from build123d import *

# Parameters (mm, degrees)
SKETCH007_R                          = 3.25
EXTRUDE006_DEPTH                     = 10
SKETCH006_AS_DRAWN_R                 = 9
EXTRUDE005_DEPTH                     = 27
EXTRUDE005_ONTO_SKETCH006_ROLL_ANGLE = 90
SKETCH_R                             = 3.5
SKETCH_R_2                           = 1.75
EXTRUDE_DEPTH                        = 30
SKETCH001_AS_DRAWN_R                 = 12.5
EXTRUDE004_DEPTH                     = 50
EXTRUDE004_ONTO_SKETCH001_ROLL_ANGLE = 90
EXTRUDE002_DEPTH                     = 60
SKETCH003_AS_DRAWN_W                 = 50
SKETCH003_AS_DRAWN_H                 = 16
EXTRUDE003_DEPTH                     = 98
EXTRUDE003_ONTO_SKETCH003_ROLL_ANGLE = 90
CHAMFER_SIZE                         = 0.5


with BuildPart() as extrude006:
    # Sketch007 → Extrude006 (new body)
    with BuildSketch(Plane.XY):
        with Locations((-16, 45)):
            Circle(SKETCH007_R)
        with Locations((16, 45)):
            Circle(SKETCH007_R)
        with Locations((-16, 65)):
            Circle(SKETCH007_R)
        with Locations((16, 65)):
            Circle(SKETCH007_R)
    extrude(amount=EXTRUDE006_DEPTH)


with BuildPart() as extrude006_1:
    # Extrude006 placement: moved
    add(extrude006.part.moved(Location((0, 0, 7))))


with BuildPart() as extrude005:
    # Sketch006 as drawn → Extrude005 (new)
    with BuildSketch(Plane.XY):
        Circle(SKETCH006_AS_DRAWN_R)
    extrude(amount=-EXTRUDE005_DEPTH)


with BuildPart() as extrude005_1:
    # Extrude005 onto Sketch006 roll: moved
    add(extrude005.part.rotate(Axis((0, 0, 0), (1, 0, 0)), EXTRUDE005_ONTO_SKETCH006_ROLL_ANGLE))


with BuildPart() as extrude005_2:
    # Extrude005 onto Sketch006 placement: moved
    add(extrude005_1.part.moved(Location((0, 33, 0))))


with BuildPart() as extrude005_3:
    # Extrude005 placement: moved
    add(extrude005_2.part.moved(Location((0, -18, 0))))


with BuildPart() as sweep_body:
    # Sweep: sweep along a path in Sketch005
    with BuildLine(Plane.YZ) as sweep_path:
        Line((70, 40), (40, 40))
        Line((40, 40), (32.928932, 47.071068))
    # Sketch004 → Sweep (sweep)
    with BuildSketch(Plane.XZ.offset(-70)):
        Polygon((-12, 16), (12, 16), (14, 10), (21, 10), (21, 28), (-21, 28), (-21, 10), (-14, 10), align=None)
    sweep(path=sweep_path.line, transition=Transition.RIGHT)


with BuildPart() as extrude_body:
    # Sketch → Extrude (new body)
    with BuildSketch(Plane.XY):
        Circle(SKETCH_R)
        with Locations((-16, 45)):
            Circle(SKETCH_R_2)
        with Locations((-16, 65)):
            Circle(SKETCH_R_2)
        with Locations((16, 65)):
            Circle(SKETCH_R_2)
        with Locations((16, 45)):
            Circle(SKETCH_R_2)
        with BuildLine():
            ThreePointArc((-12.020815, -9.192388), (-12.020815, -12.020815), (-9.192388, -12.020815))
            Line((-9.192388, -12.020815), (-4.242641, -7.071068))
            ThreePointArc((-4.242641, -7.071068), (-4.242641, -4.242641), (-7.071068, -4.242641))
            Line((-12.020815, -9.192388), (-7.071068, -4.242641))
        make_face()
        with BuildLine():
            ThreePointArc((7.071068, -4.242641), (4.242641, -4.242641), (4.242641, -7.071068))
            Line((4.242641, -7.071068), (9.192388, -12.020815))
            ThreePointArc((9.192388, -12.020815), (12.020815, -12.020815), (12.020815, -9.192388))
            Line((7.071068, -4.242641), (12.020815, -9.192388))
        make_face()
        with BuildLine():
            ThreePointArc((4.242641, 7.071068), (4.242641, 4.242641), (7.071068, 4.242641))
            Line((7.071068, 4.242641), (12.020815, 9.192388))
            ThreePointArc((12.020815, 9.192388), (12.020815, 12.020815), (9.192388, 12.020815))
            Line((4.242641, 7.071068), (9.192388, 12.020815))
        make_face()
        with BuildLine():
            ThreePointArc((-9.192388, 12.020815), (-12.020815, 12.020815), (-12.020815, 9.192388))
            Line((-12.020815, 9.192388), (-7.071068, 4.242641))
            ThreePointArc((-7.071068, 4.242641), (-4.242641, 4.242641), (-4.242641, 7.071068))
            Line((-9.192388, 12.020815), (-4.242641, 7.071068))
        make_face()
        with BuildLine():
            ThreePointArc((6.4, 17.2), (0, 30), (-6.4, 17.2))
            Line((-6.4, 17.2), (-1.6, 10.8))
            ThreePointArc((-1.6, 10.8), (0, 10), (1.6, 10.8))
            Line((6.4, 17.2), (1.6, 10.8))
        make_face()
        with BuildLine():
            ThreePointArc((-21, 11.61895), (0, -24), (21, 11.61895))
            Line((21, 70), (21, 11.61895))
            Line((30, 70), (21, 70))
            Line((30, -30), (30, 70))
            Line((-30, -30), (30, -30))
            Line((-30, 70), (-30, -30))
            Line((-21, 70), (-30, 70))
            Line((-21, 11.61895), (-21, 70))
        make_face()
    extrude(amount=EXTRUDE_DEPTH)


with BuildPart() as extrude004:
    # Sketch001 as drawn → Extrude004 (new)
    with BuildSketch(Plane.XY):
        Circle(SKETCH001_AS_DRAWN_R)
    extrude(amount=-EXTRUDE004_DEPTH)


with BuildPart() as extrude004_1:
    # Extrude004 onto Sketch001 roll: moved
    add(extrude004.part.rotate(Axis((0, 0, 0), (1, 0, 0)), EXTRUDE004_ONTO_SKETCH001_ROLL_ANGLE))


with BuildPart() as extrude004_2:
    # Extrude004 onto Sketch001 placement: moved
    add(extrude004_1.part.moved(Location((0, 32, 0))))


with BuildPart() as extrude002:
    # Sketch002 → Extrude002 (new body)
    with BuildSketch(Plane.YZ.offset(33)):
        Polygon((-30, 9), (15, 9), (24, 0), (-30, 0), align=None)
    extrude(amount=-EXTRUDE002_DEPTH)


with BuildPart() as chamfer_body:
    # Sketch003 as drawn → Extrude003 (new)
    with BuildSketch(Plane.XY):
        with Locations((0, 8)):
            Rectangle(SKETCH003_AS_DRAWN_W, SKETCH003_AS_DRAWN_H)
    extrude(amount=-EXTRUDE003_DEPTH)


with BuildPart() as chamfer_body_1:
    # Extrude003 onto Sketch003 roll: moved
    add(chamfer_body.part.rotate(Axis((0, 0, 0), (1, 0, 0)), EXTRUDE003_ONTO_SKETCH003_ROLL_ANGLE))


with BuildPart() as chamfer_body_2:
    # Extrude003 onto Sketch003 placement: moved
    add(chamfer_body_1.part.moved(Location((0, -28, 0))))

    # Cut: cut Extrude002
    add(extrude002.part, mode=Mode.SUBTRACT)

    # Cut001: cut Extrude004
    add(extrude004_2.part, mode=Mode.SUBTRACT)

    # Cut002: cut Extrude body
    add(extrude_body.part, mode=Mode.SUBTRACT)

    # Cut003: cut Sweep body
    add(sweep_body.part, mode=Mode.SUBTRACT)

    # Cut004: cut Extrude005
    add(extrude005_3.part, mode=Mode.SUBTRACT)

    # Cut005: cut Extrude006
    add(extrude006_1.part, mode=Mode.SUBTRACT)

    # Chamfer
    chamfer_edges = [chamfer_body_2.edges().sort_by_distance(p)[0] for p in [
        (12.5, 51, 0),
        (0, 70, 12.5),
        (-12.5, 51, 0),
    ]]
    chamfer(chamfer_edges, length=CHAMFER_SIZE)


solid = chamfer_body_2.part
Work out the finished part from the listing and answer in its coordinate system (mm). A direction names the side the tool comes from. Give positions to 0.01 mm unless a question says otherwise; leave off trailing zeros. Order: outer loops, then holes, each group sorted by start corner. A loop starts at its lowest first (then second) coordinate and runs counter-clockwise, first axis right, second up. Notation, with made-up numbers: (34, 51.25) - (49, 51.25) arc R28 ccw to (49, 79.25) - close; hole circle Ø4 at (22.5, 88.25). An arc over 180 degrees is marked (long way). Answer as CSV lines item,"result". Start each with the question number.
Q1. The mould has two halves that part along X. Classify faces 4 (the face through (11.99, -12.05, 12.45)), 5 (the face through (5, 12, 16)), 6 (the face through (21, 41, 6)): +X half, -X half, draft (parallel to the pull), parting line (faces both ways), or undercut.
Q2. The part is cut by section A-A (x = 0). Write down the section's boundary in (y, z).
Q3. Find the intervals of material crossed by L1, parallel to X at y = 45, z = 3.5; L2, parallel to Y at x = 16, z = 4.5; L3, parallel to Y at x = 16, z = 4.25, in increasing order. Write a range as [from, to].
Q4. The part is cut by section B-B (y = 45). Write down the section's boundary in (x, z), then the cut area to 3 significant figures.
Q5. Given pin 1 Ø3.5 at (x, y) = (-18.5, 53) entering from +Z; pin 2 Ø4.5 at (x, y) = (16, 65) entering from +Z; pin 3 Ø5 at (x, z) = (-9, 6) entering from +Y; pin 4 Ø8 at (y, z) = (-8.5, 13.5) entering from -X, each flat-ended and moving along its own axis, determine where each tip first touches the part or whether it passes through.
Q6. The part is cut by section C-C (y = 31). Write down the section's boundary in (x, z), then the cut area to 3 significant figures.
Q7. The part is cut by section D-D (z = 3.25). Give the number of separate pieces and of enclosed holes in the cut face, then the cut area to 3 significant figures.
Q8. For faces 1 (the face through (-18, 48, 10)), 2 (the face through (0, -5, 9)), 3 (the face through (4, 14, 12)), determine the directions among +Z, -Z, +X, -X, +Y, -Y from which every point of the face is accessible in a straight line to the end or side of a thin tool.
Check result:
1,face 4,"undercut"
1,face 5,"draft"
1,face 6,"+X half"
2,outline,"(-24, 9) - (-3.5, 9) - (-3.5, 16) - (-24, 16) - close; (3.5, 9) - (10, 9) - (10, 16) - (3.5, 16) - close; (30, 9) - (32, 9) - (32, 12.5) - (69.5, 12.5) - (70, 13) - (70, 16) - (30, 16) - close"
3,L1,"x = [-21, -17.75], [-14.25, -12], [12, 14.25], [17.75, 21]"
3,L2,"y = [19.5, 43.25], [46.75, 63.25], [66.75, 70]"
3,L3,"y = [19.75, 43.25], [46.75, 63.25], [66.75, 70]"
4,outline,"(-21, 0) - (-17.75, 0) - (-17.75, 7) - (-19.25, 7) - (-19.25, 10) - (-21, 10) - close; (-14.25, 0) - (-13, 0) - (-12.49, 0.5) arc R12.5 cw to (12.49, 0.5) - (13, 0) - (14.25, 0) - (14.25, 7) - (12.75, 7) - (12.75, 13.75) - (12, 16) - (-12, 16) - (-12.75, 13.75) - (-12.75, 7) - (-14.25, 7) - close; (17.75, 0) - (21, 0) - (21, 10) - (19.25, 10) - (19.25, 7) - (17.75, 7) - close"
4,area,"238 mm²"
5,pin 1,"stops at z = 10"
5,pin 2,"stops at z = 7"
5,pin 3,"stops at y = 70"
5,pin 4,"stops at x = -23.57"
6,outline,"(-21, 0) - (-9, 0) arc R9 cw to (9, 0) - (21, 0) - (21, 10) - (14, 10) - (12, 16) - (-12, 16) - (-14, 10) - (-21, 10) - close"
6,area,"449 mm²"
7,separate pieces,"2"
7,enclosed holes,"4"
7,area,"924 mm²"
8,face 1,"+Z, -X, +Y"
8,face 2,"-Z, +X, -X, -Y"
8,face 3,"+Z, -Z"
